Check sheet for the drawn part. Datum: minimum x, y, z corner. Units: mm. A direction names the side the tool comes from. Give positions to 0.01 mm unless a question says otherwise; leave off trailing zeros. Order: outer loops, then holes, each group sorted by start corner. A loop starts at its lowest first (then second) coordinate and runs counter-clockwise, first axis right, second up.
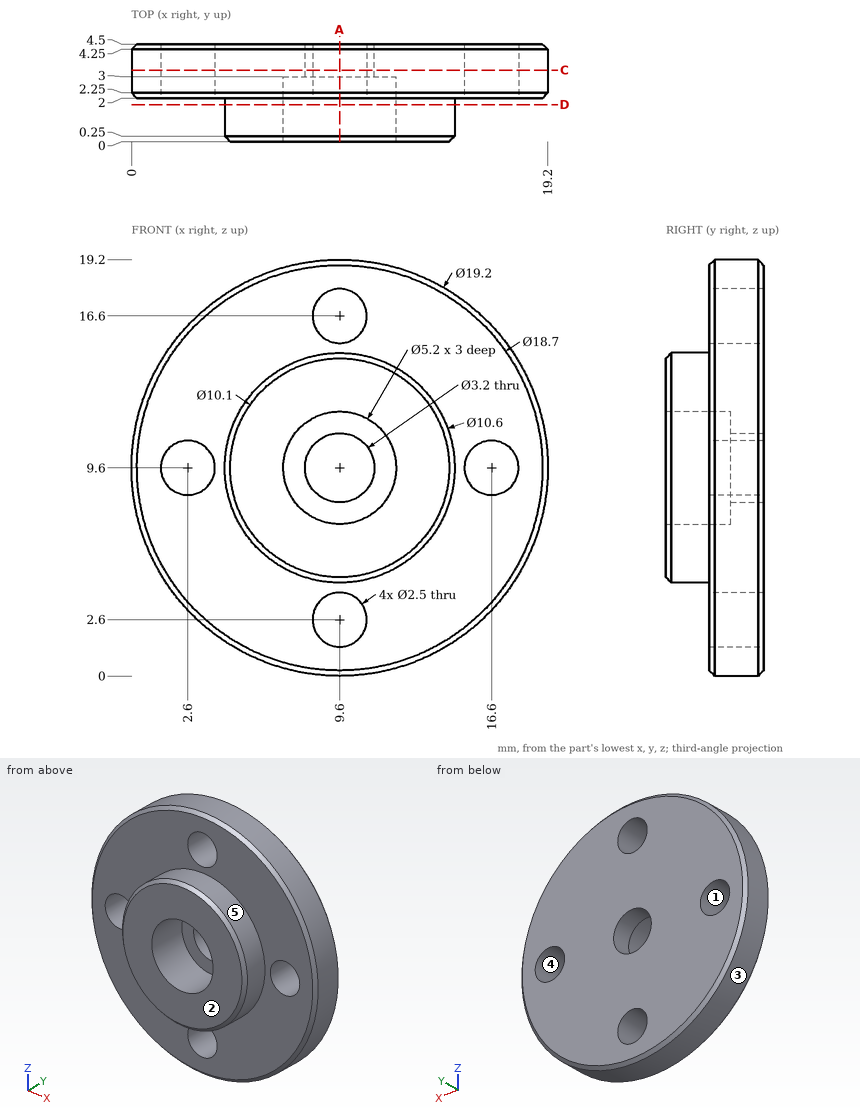
(1) Section check A-A, the plane x = 9.6. Give the number of separate pieces and of enclosed holes in the cut face, then the cut area to 3 significant figures.
Solved:
separate pieces: 4
enclosed holes: 0
area: 36.1 mm2
(2) Section check D-D, the plane y = 1.7. Enter the section's corners in (x, z), then the cut area to 3 significant figures.
Solved:
outline: circle Ø10.6 at (9.6, 9.6); hole circle Ø5.2 at (9.6, 9.6)
area: 67.0 mm2
(3) Section check C-C, the plane y = 3.3. Enter the section's corners in (x, z), then the cut area to 3 significant figures.
Solved:
outline: circle Ø19.2 at (9.6, 9.6); hole circle Ø2.5 at (2.6, 9.6); hole circle Ø3.2 at (9.6, 9.6); hole circle Ø2.5 at (9.6, 2.6); hole circle Ø2.5 at (9.6, 16.6); hole circle Ø2.5 at (16.6, 9.6)
area: 262 mm2
(4) Set-up check for the marked faces 4 and 5: record each of +Z, -Z, +X, -X, +Y, -Y from which the full face is reachable in a straight line by a thin tool's end or side.
Solved:
face 4: +Y, -Y
face 5: -Y
(5) Scan lines: line 1 (X direction, y = 3.4, z = 9.6); line 2 (Z direction, x = 9, y = 4); line 3 (Z direction, x = 8.5, y = 3.4). Record each from-to range of solid material in increasing order.
Solved:
line 1: x = 0 to 1.35, 3.85 to 8, 11.2 to 15.35, 17.85 to 19.2
line 2: z = 0.02 to 1.5, 3.7 to 8.12, 11.08 to 15.5, 17.7 to 19.18
line 3: z = 0.06 to 2.01, 3.19 to 8.44, 10.76 to 16.01, 17.19 to 19.14
(6) Go/stop test with flat-tipped pins: pin 1 (1.6 mm diameter, centred on x = 10.5, z = 9.5, fed in from -Y); pin 2 (1.5 mm diameter, centred on x = 8, y = 1, fed in from +Z); pin 3 (4 mm diameter, centred on x = 7.5, z = 2, fed in from -Y). Record where each tip stops, or that it passes through.
Solved:
pin 1: stops at y = 3
pin 2: stops at z = 14.83
pin 3: stops at y = 2
(7) Release check for a two-part mould opening along X. For the marked faces 1, 2 and 3 record: pulls with the +X half, pulls with the -X half, needs draft (parallel to the pull), parting line crosses it, or undercut.
Solved:
face 1: undercut
face 2: needs draft
face 3: parting line crosses it
